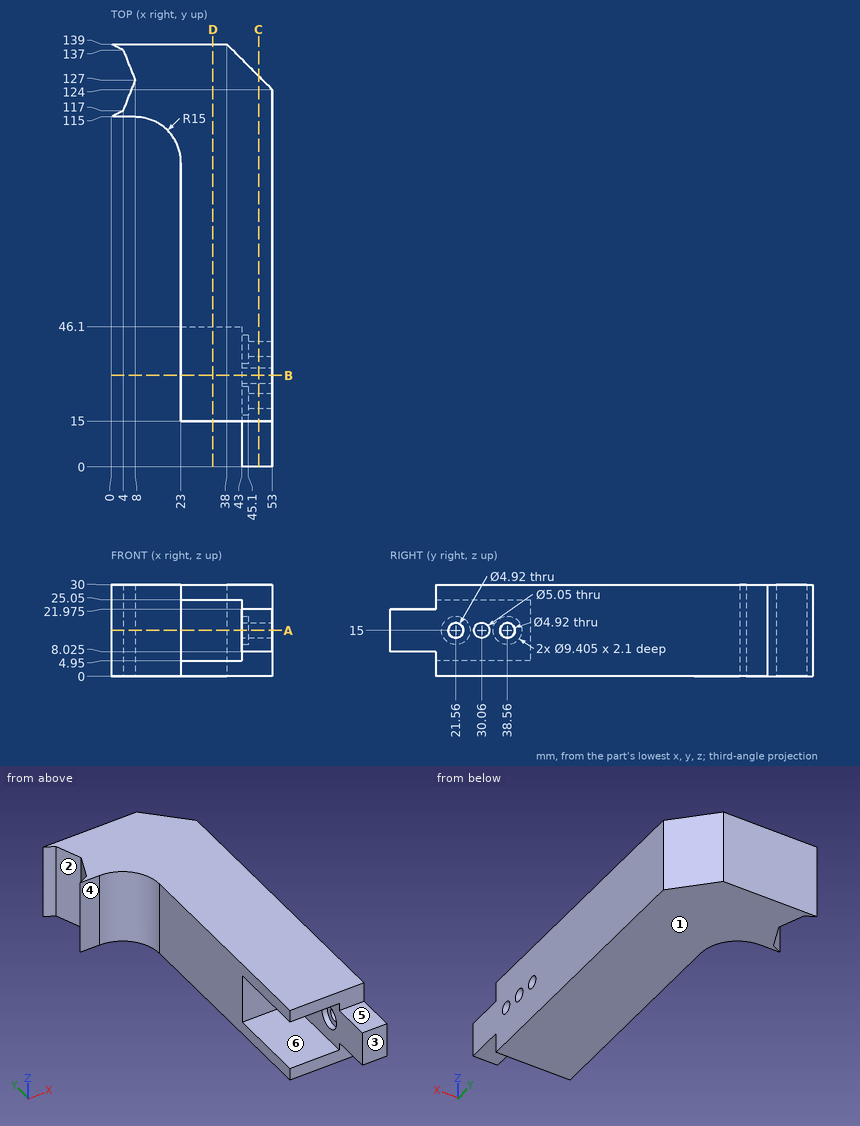
Design review of the part shown in the three views and the two pictorial views. Dimensions are in mm from the part's minimum x, y and z. A direction names the side the tool comes from. Round coordinates to 2 decimals unless told otherwise and drop trailing zeros. Loops run counter-clockwise (first coordinate to the right, second up) from the corner with the lowest first, then second, coordinate; pieces in that order, holes last. Notation, with made-up numbers: (5.25, 52) - (61.25, 52) arc R25 ccw to (61.25, 66) - close; hole circle Ø6 at (-29, -1.75). An arc over 180 degrees is marked (long way). Use one line per item in the form item = value.
1) We need section D-D on x = 33.5. Write out the cut boundary in (y, z).
Solutions:
outline = (15, 0) - (139, 0) - (139, 30) - (15, 30) - (15, 25.05) - (46.1, 25.05) - (46.1, 4.95) - (15, 4.95) - close
2) We need section A-A on z = 15. State how many separate pieces and enclosed holes the cut face has, then the cut area to 3 significant figures.
Solutions:
separate_pieces = 4
enclosed_holes = 0
area = 3,440 mm2
3) Mouldability with a two-part tool opening along Y and no side actions: class the marked faces 1, 2 and 3 as pulls with the +Y half, pulls with the -Y half, needs draft (parallel to the pull), parting line crosses it, or undercut.
Solutions:
face_1 = needs draft
face_2 = undercut
face_3 = pulls with the -Y half
4) Wall thickness on probe 1 along Z at (x, y) = (47.25, 21.56); probe 2 along Y at (x, z) = (44.4, 15) (1 decimal); probe 3 along X at (y, z) = (67.5, 14.5): over which ranges is each line inside the solid? List them lowest first.
Solutions:
probe_1 = 0 to 12.54, 17.46 to 30
probe_2 = 0 to 16.9, 26.3 to 27.5, 32.6 to 33.9, 43.3 to 132.6
probe_3 = 23 to 53
5) We need section C-C on x = 48.5. Write out the cut boundary in (y, z) (3 decimals).
Solutions:
outline = (0, 8.025) - (15, 8.025) - (15, 0) - (128.5, 0) - (128.5, 30) - (15, 30) - (15, 21.975) - (0, 21.975) - close; hole circle Ø4.92 at (21.56, 15); hole circle Ø5.05 at (30.06, 15); hole circle Ø4.92 at (38.56, 15)
6) Tool access review of the marked faces 4, 5 and 6: name each direction out of +Z, -Z, +X, -X, +Y, -Y from which nothing blocks a thin tool from reaching the whole face with its end or side.
Solutions:
face_4 = +Z, -Z, -X, -Y
face_5 = +Z, +X, -X, -Y
face_6 = -X, -Y
7) We need section B-B on y = 30.06. Write out the cut boundary in (x, z) (3 decimals), then the cut area to 4 significant figures.
Solutions:
outline = (23, 0) - (53, 0) - (53, 12.475) - (43, 12.475) - (43, 4.95) - (23, 4.95) - close; (23, 25.05) - (43, 25.05) - (43, 17.525) - (53, 17.525) - (53, 30) - (23, 30) - close
area = 447.5 mm2
8) Clearance check with flat-ended pins moving along their axes: P1, Ø10.5, axis at y = 22.5, z = 13, coming from the -X side; P2, Ø3, axis at y = 30.06, z = 15, coming from the -X side; P3, Ø7.5, axis at y = 38.56, z = 15, coming from the -X side; P4, Ø8, axis at x = 49, y = 5.5, coming from the -Z side (3 decimals). State where each tip first meets the part, or that it passes through.
Solutions:
P1 = 43
P2 = through
P3 = 45.1
P4 = 8.025
